Input: part model. Units: mm. Frame: model coordinates. A direction names the side the tool comes from. Give positions to 0.01 mm unless a question says otherwise; leave off trailing zeros. Loops run counter-clockwise (first coordinate to the right, second up) from the corner with the lowest first, then second, coordinate; pieces in that order, holes last. Notation, with made-up numbers: (16, 77.25) -> (26, 77.25) arc R25 cw to (26, 103.25) -> close; hole circle Ø2 at (-28, 56). An arc over 180 degrees is marked (long way). Answer as a JSON object with one key per item and string values.
```python
from build123d import *

# Parameters (mm, degrees)
SKIZZE1_R                       = 26.5
AUFSATZ_LINEAR_AUSTRAGEN1_DEPTH = 5
SKIZZE2_W                       = 5.565713714
SKIZZE2_H                       = 5
AUFSATZ_LINEAR_AUSTRAGEN2_DEPTH = 6
DURCHGANGSLOCH_F_R_M21_D        = 2.4


with BuildPart() as part:
    # Skizze1 → Aufsatz-Linear austragen1 (new body)
    with BuildSketch(Plane.XY):
        with BuildLine():
            Line((70.565713714, 5), (64.565713714, 5))
            ThreePointArc((64.565713714, 5), (35.493867542, 28.995582938), (7.277186767, 4))
            ThreePointArc((7.277186767, 4), (-0.001790997, 7.744118326), (-7.275862069, 3.990476177))
            ThreePointArc((-7.275862069, 3.990476177), (-35.489060527, 28.995498631), (-64.565713714, 5))
            Line((-64.565713714, 5), (-70.565713714, 5))
            Line((-70.565713714, 5), (-70.565713714, 0))
            Line((-70.565713714, 0), (-65, 0))
            ThreePointArc((-65, 0), (-36, -29), (-7, 0))
            ThreePointArc((-7, 0), (0, 4.807417596), (7, 0))
            ThreePointArc((7, 0), (36, -29), (65, 0))
            Line((65, 0), (70.565713714, 0))
            Line((70.565713714, 0), (70.565713714, 5))
        make_face()
        with Locations((36, 0)):
            Circle(SKIZZE1_R, mode=Mode.SUBTRACT)
        with Locations((-36, 0)):
            Circle(SKIZZE1_R, mode=Mode.SUBTRACT)
    extrude(amount=AUFSATZ_LINEAR_AUSTRAGEN1_DEPTH)

    # Skizze2 → Aufsatz-Linear austragen2 (add)
    with BuildSketch(Plane(origin=(0, 0, 0), x_dir=(-1, 0, 0), z_dir=(0, 0, -1))):
        with Locations((-67.782856857, 2.5)):
            Rectangle(SKIZZE2_W, SKIZZE2_H)
        with Locations((67.782856857, 2.5)):
            Rectangle(SKIZZE2_W, SKIZZE2_H)
    extrude(amount=AUFSATZ_LINEAR_AUSTRAGEN2_DEPTH)

    # Durchgangsloch für M21 (through all)
    with Locations(Plane(origin=(0, 5, 0), x_dir=(1, 0, 0), z_dir=(0, 1, 0))):
        with Locations((-67.815713714, 3), (67.815713714, 3)):
            Hole(DURCHGANGSLOCH_F_R_M21_D / 2)


solid = part.part
```
Q1. Draft query along Y for faces 4 (the flat face through (68, 5, 0)), 5 (the flat face through (-68, 3, -6)), 6 (the cylindrical face through (-62.474, 1.165, 2.465)). Return one class per face: +Y half, -Y half, draft (parallel to the pull), parting line (faces both ways), or undercut.
Evaluation:
{"face 4": "+Y half", "face 5": "draft", "face 6": "undercut"}
Q2. Pin query (flat end, axial travel): pin 1 (5 mm diameter, centred on y = -12.5, z = 0.5, fed in from -X); pin 2 (1 mm diameter, centred on y = -6.5, z = 4, fed in from -X); pin 3 (1.5 mm diameter, centred on y = -2.5, z = 1, fed in from +X). Return the tip coordinate at first contact, or that it passes through.
Evaluation:
{"pin 1": "stops at x = -63.22", "pin 2": "stops at x = -64.37", "pin 3": "stops at x = 64.95"}
Q3. Ray query, line 1 along X through (y, z) = (-17, 4); line 2 along Y through (x, z) = (36, 1.2); line 3 along X through (y, z) = (-20, 1.75). Return the intervals inside material, ascending.
Evaluation:
{"line 1": "x = -59.49 to -56.33, -15.67 to -12.51, 12.51 to 15.67, 56.33 to 59.49", "line 2": "y = -29 to -26.5, 26.5 to 29", "line 3": "x = -57 to -53.39, -18.61 to -15, 15 to 18.61, 53.39 to 57"}
Q4. Section A-A, the plane x = -36. Return the cut outline in (y, z), then the cut area to 3 significant figures.
Evaluation:
{"outline": "(-29, 0) -> (-26.5, 0) -> (-26.5, 5) -> (-29, 5) -> close; (26.5, 0) -> (29, 0) -> (29, 5) -> (26.5, 5) -> close", "area": "25.0 mm2"}
Q5. Section B-B, the plane z = 2.25. Return the cut outline in (x, y), then the cut area to 3 significant figures.
Evaluation:
{"outline": "(-70.57, 0) -> (-65, 0) arc R29 ccw to (-7, 0) arc R7.5 cw to (7, 0) arc R29 ccw to (65, 0) -> (70.57, 0) -> (70.57, 5) -> (64.57, 5) arc R29 ccw to (7.28, 4) arc R8.94 ccw to (-7.28, 3.99) arc R29 ccw to (-64.57, 5) -> (-70.57, 5) -> close; hole circle Ø53 at (-36, 0); hole circle Ø53 at (36, 0)", "area": "975 mm2"}
Q6. Section D-D, the plane x = 48.5. Return the cut outline in (y, z), then the cut area to 3 significant figures.
Evaluation:
{"outline": "(-26.17, 0) -> (-23.37, 0) -> (-23.37, 5) -> (-26.17, 5) -> close; (23.37, 0) -> (26.17, 0) -> (26.17, 5) -> (23.37, 5) -> close", "area": "28.0 mm2"}
Q7. Access query for faces 1 (the cylindrical face through (35.362, -28.993, 2.465)), 2 (the flat face through (-68, 0, -1)), 3 (the flat face through (-68, 5, -1)). Directions: +Z, -Z, +X, -X, +Y, -Y. A direction counts if a zero-diameter tool reaches every point of the face in a straight line with its end or side. Return the directions, or none.
Evaluation:
{"face 1": "+Z, -Z, -Y", "face 2": "+Z, -Z, -X, -Y", "face 3": "+Z, -Z, -X, +Y"}
Q8. Section C-C, the plane y = 13.5. Return the cut outline in (x, z).
Evaluation:
{"outline": "(-61.67, 0) -> (-58.8, 0) -> (-58.8, 5) -> (-61.67, 5) -> close; (-13.2, 0) -> (-10.33, 0) -> (-10.33, 5) -> (-13.2, 5) -> close; (10.33, 0) -> (13.2, 0) -> (13.2, 5) -> (10.33, 5) -> close; (58.8, 0) -> (61.67, 0) -> (61.67, 5) -> (58.8, 5) -> close"}
